Here's the drawing with two shaded views (mm, measured from the low corner). I have some questions. A direction names the side the tool comes from. Coordinates: 2 decimals unless noted, no trailing zeros. Loops run counter-clockwise (first coordinate to the right, second up) from the corner with the lowest first, then second, coordinate; pieces in that order, holes last. Notation, with made-up numbers: (-37, 68) - (0, 68) arc R10 ccw to (0, 76) - close; hole circle Ø11 at (65.25, -39.75). An arc over 180 degrees is marked (long way). One line per item, written item: value. Start each with the question number.
(1) If we section it at C-C on x = 52: Write out the boundary of the cut face in (y, z).
(2) On a 3-axis mill with a long thin cutter (end or side, diameter ignored), from which of +Z, -Z, +X, -X, +Y, -Y can I reach the whole of each face in a straight line? I mean the marked faces 4 and 5. Say none if no direction works.
(3) If I drill on line 1 along X through (y, z) = (5, 5); line 2 along X through (y, z) = (3.5, 10.5); line 3 along X through (y, z) = (5.75, 6), over which ranges is the centre line in solid material (lowest first)? Write a range as from..to.
(4) If we mould it in two halves opening along X, with no side actions, what happens to the marked faces 1, 2 and 3? For each: pulls with the +X half, pulls with the -X half, needs draft (parallel to the pull), parting line crosses it, or undercut.
(5) If we section it at A-A on z = 15: Write out the boundary of the cut face in (x, y).
(6) If we section it at B-B on y = 1.75: Write out the boundary of the cut face in (x, z).
(7) If we section it at D-D on x = 36.5: Write out the boundary of the cut face in (y, z), then the cut area to 3 significant figures.
(8) I'm going to push a flat-ended pin straight in: P1, Ø1.5, axis at x = 37, y = 2.5, coming from the +Z side. Where does the tip first touch, or does it pass through?
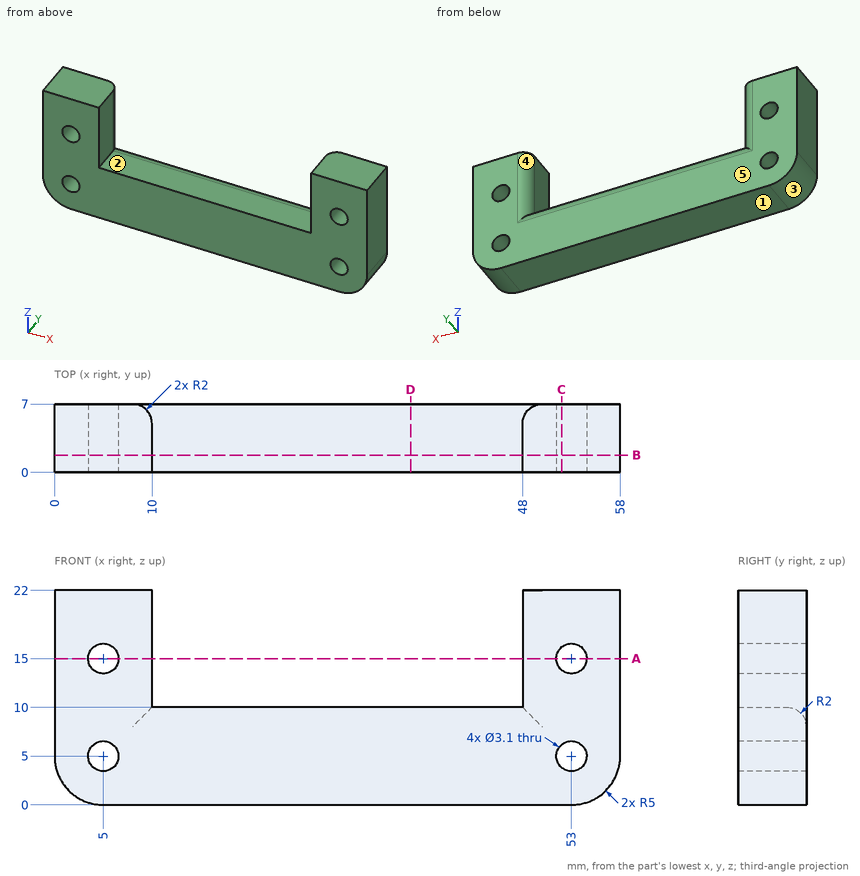
Values:
1. outline: (0, 0) - (7, 0) - (7, 3.82) - (0, 3.82) - close; (0, 6.18) - (7, 6.18) - (7, 13.82) - (0, 13.82) - close; (0, 16.18) - (7, 16.18) - (7, 22) - (0, 22) - close
2. face 4: +Z, +Y
2. face 5: +Z, -Z, +X, -X, +Y
3. line 1: x = 0..3.45, 6.55..51.45, 54.55..58
3. line 2: x = 0..10, 48..58
3. line 3: x = 0..3.82, 6.18..51.82, 54.18..58
4. face 1: needs draft
4. face 2: undercut
4. face 3: pulls with the -X half
5. outline: (0, 0) - (3.45, 0) - (3.45, 7) - (0, 7) - close; (6.55, 0) - (10, 0) - (10, 5) arc R2 ccw to (8, 7) - (6.55, 7) - close; (48, 0) - (51.45, 0) - (51.45, 7) - (50, 7) arc R2 ccw to (48, 5) - close; (54.55, 0) - (58, 0) - (58, 7) - (54.55, 7) - close
6. outline: (0, 5) arc R5 ccw to (5, 0) - (53, 0) arc R5 ccw to (58, 5) - (58, 22) - (48, 22) - (48, 10) - (10, 10) - (10, 22) - (0, 22) - close; hole circle Ø3.1 at (5, 5); hole circle Ø3.1 at (5, 15); hole circle Ø3.1 at (53, 5); hole circle Ø3.1 at (53, 15)
7. outline: (0, 0) - (7, 0) - (7, 8) arc R2 ccw to (5, 10) - (0, 10) - close
7. area: 69.1 mm2
8. P1: stops at z = 10
